Check sheet for the modelled part. Datum: model origin and axes. Units: mm. Round coordinates to 2 decimals unless told otherwise and drop trailing zeros. Loops run counter-clockwise (first coordinate to the right, second up) from the corner with the lowest first, then second, coordinate; pieces in that order, holes last. Notation, with made-up numbers: (44.5, 10) - (53.5, 10) arc R25 cw to (53.5, 23) - close; hole circle Ø8 at (-16.75, 83.25). An arc over 180 degrees is marked (long way). Put each result on its own line as item: value. Start each with the question number.
Item 1: Section check D-D, the plane z = 48. Record the cut outline in (x, y) (1 decimal).
Item 2: Section check B-B, the plane y = 0.25. Record the cut outline in (x, z) (3 decimals), and give its area (3 significant figures).
Item 3: Section check C-C, the plane z = 35.5. Record the cut outline in (x, y) (1 decimal), and give its area (3 significant figures).
Item 4: Section check A-A, the plane x = 0. Record the cut outline in (y, z), and give its area (3 significant figures).
Item 5: Gauge pin test, flat ends, axial feed: pin 1 Ø19 at (x, z) = (0, 30.26) entering from +Y; pin 2 Ø3 at (x, y) = (21.5, 3) entering from -Z. Record the tip position at first contact, or that the pin passes through.
Item 6: Material ranges on line 1 along Y through (x, z) = (5.5, 9); line 2 along X through (y, z) = (-0.25, 51.5) (3 decimals); line 3 along Z through (x, y) = (-16, 0.5), recorded low to high.
from build123d import *

# Parameters (mm, degrees)
F0_W     = 57.15
F0_H     = 9.779
F0_W_2   = 50.8
F0_H_2   = 3.429
F1_DEPTH = 57.15
F2_DEPTH = 6.35
F3_R     = 15.875
F4_DEPTH = 9.78


with BuildPart() as f1:
    # F0 (on Top) → F1 (new body)
    with BuildSketch(Plane.XY):
        Rectangle(F0_W, F0_H)
        Rectangle(F0_W_2, F0_H_2, mode=Mode.SUBTRACT)
    extrude(amount=F1_DEPTH)

    # F0 (on Top) → F2 (join)
    with BuildSketch(Plane.XY):
        Rectangle(F0_W_2, F0_H_2)
    extrude(amount=F2_DEPTH)

    # F3 (on face) → F4 (cut, through all)
    with BuildSketch(Plane.XZ.offset(4.8895)):
        with Locations((0, 30.261343)):
            Circle(F3_R)
    extrude(amount=-F4_DEPTH, mode=Mode.SUBTRACT)


solid = f1.part
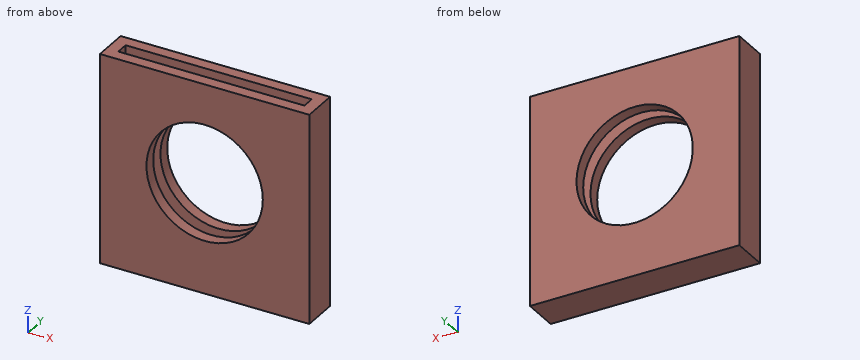
Check result:
1. outline: (-28.6, -4.9) - (28.6, -4.9) - (28.6, 4.9) - (-28.6, 4.9) - close; hole (-25.4, -1.7) - (25.4, -1.7) - (25.4, 1.7) - (-25.4, 1.7) - close
2. outline: (-28.575, 0) - (28.575, 0) - (28.575, 57.15) - (25.4, 57.15) - (25.4, 6.35) - (-25.4, 6.35) - (-25.4, 57.15) - (-28.575, 57.15) - close
2. area: 685 mm²
3. outline: (-28.6, -4.9) - (-15, -4.9) - (-15, -1.7) - (-25.4, -1.7) - (-25.4, 1.7) - (-15, 1.7) - (-15, 4.9) - (-28.6, 4.9) - close; (15, -4.9) - (28.6, -4.9) - (28.6, 4.9) - (15, 4.9) - (15, 1.7) - (25.4, 1.7) - (25.4, -1.7) - (15, -1.7) - close
3. area: 194 mm²
4. outline: (-4.89, 0) - (4.89, 0) - (4.89, 14.39) - (1.71, 14.39) - (1.71, 6.35) - (-1.71, 6.35) - (-1.71, 14.39) - (-4.89, 14.39) - close; (-4.89, 46.14) - (-1.71, 46.14) - (-1.71, 57.15) - (-4.89, 57.15) - close; (1.71, 46.14) - (4.89, 46.14) - (4.89, 57.15) - (1.71, 57.15) - close
4. area: 183 mm²
5. pin 1: through
5. pin 2: z = 0
6. line 1: -4.89 to -1.71, 1.71 to 4.89
6. line 2: -28.575 to -25.4, 25.4 to 28.575
6. line 3: 0 to 6.35
